Input: dimensioned drawing with shaded views. Units: mm. Origin: part minimum x, y, z. A direction names the side the tool comes from. Round coordinates to 2 decimals unless told otherwise and drop trailing zeros. Loops run counter-clockwise (first coordinate to the right, second up) from the corner with the lowest first, then second, coordinate; pieces in that order, holes last. Notation, with made-up numbers: (48.5, 47.5) - (54.5, 47.5) arc R23 ccw to (54.5, 56.5) - close; hole circle Ø1 at (-19.75, 78.25). An arc over 180 degrees is marked (long way). Answer as a JSON object with one key per item and string values. Group by question number.
Item 1: Section B-B (z = 5.75). Return the cut outline in (x, y) (3 decimals), plus the area to 3 significant figures.
Item 2: Reachability of the marked faces 1 and 2 from +Z, -Z, +X, -X, +Y, -Y: full face, straight path, thin tool, end or side. Return the list, or none.
Item 3: First-contact query: pin 1 (3 mm diameter, centred on x = 9.5, z = 2, fed in from +Y). Flat tip, straight axial feed; report the tip coordinate or a pass-through.
Item 4: Section A-A (z = 1.5). Return the cut outline in (x, y), plus the area to 3 significant figures.
Item 5: Line query: line 1 (Z direction, x = 4, y = 11); line 2 (Y direction, x = 13, z = 1); line 3 (X direction, y = 13.25, z = 6). Output: solid intervals per line, ascending.
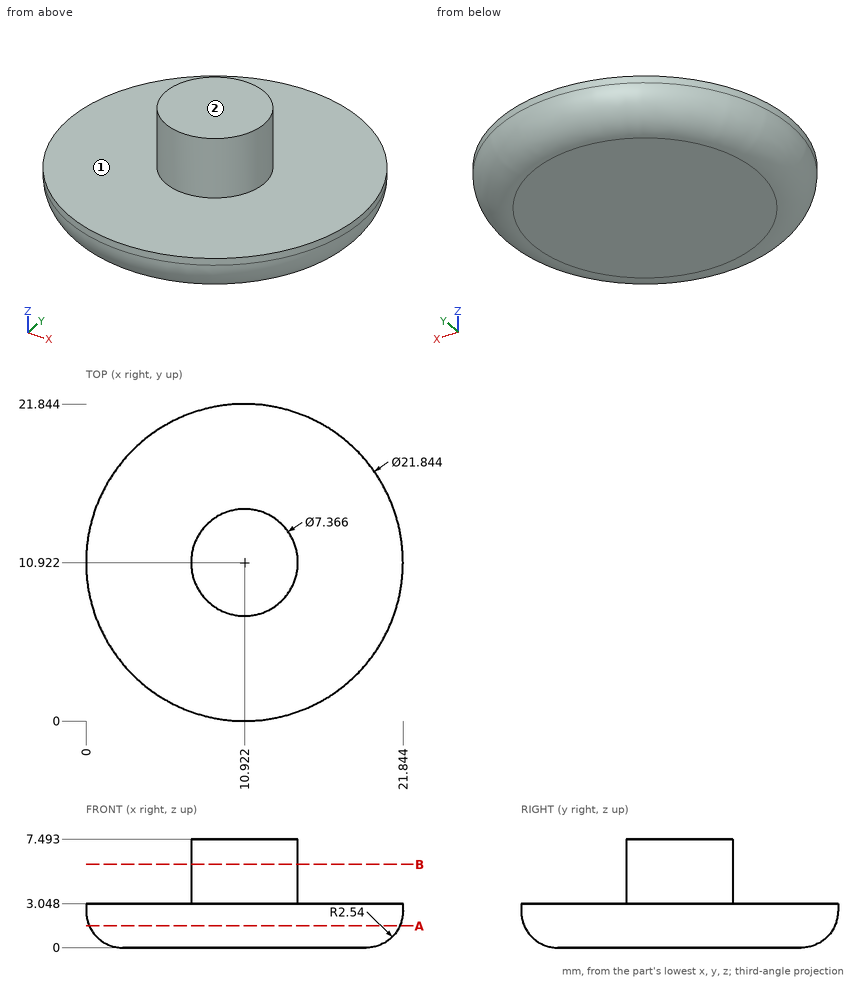
Values:
{
 "1": {"outline": "circle Ø7.366 at (10.922, 10.922)", "area": "42.6 mm^2"},
 "2": {"face 1": "+Z", "face 2": "+Z, +X, -X, +Y, -Y"},
 "3": {"pin 1": "stops at y = 21.84"},
 "4": {"outline": "circle Ø21.4 at (10.92, 10.92)", "area": "360 mm^2"},
 "5": {"line 1": "z = 0 to 3.05", "line 2": "y = 0.73 to 21.11", "line 3": "x = 8.07 to 13.78"}
}
